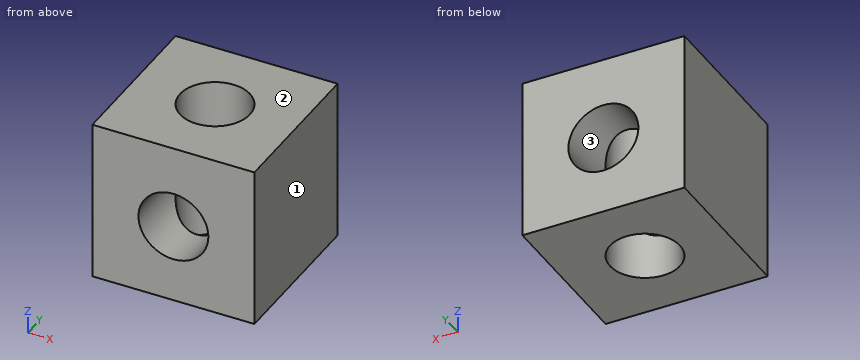
from build123d import *

# Parameters (mm, degrees)
F0_W     = 44.704
F0_H     = 44.704
F0_R     = 9.652
F1_DEPTH = 43.688
F2_R     = 9.652
F3_DEPTH = 44.705


with BuildPart() as f1:
    # F0 (on Front) → F1 (new body)
    with BuildSketch(Plane.XZ):
        with Locations((-17.125217, 3.559626)):
            Rectangle(F0_W, F0_H)
        with Locations((-17.125217, 2.924626)):
            Circle(F0_R, mode=Mode.SUBTRACT)
    extrude(amount=F1_DEPTH)

    # F2 (on face) → F3 (cut, through all)
    with BuildSketch(Plane.XY.offset(25.911626)):
        with Locations((-17.125217, -21.844)):
            Circle(F2_R)
    extrude(amount=-F3_DEPTH, mode=Mode.SUBTRACT)


solid = f1.part
Can you work these out from the model? Positions are in its coordinate system, mm. Face numbers are marked on the shaded views. Coordinates: 2 decimals unless noted, no trailing zeros. Write each loop counter-clockwise with the first axis right and the second up, starting at its lowest first coordinate (ties: lowest second). Pieces come first, ordered by that corner, then holes. Notation, with made-up numbers: (81, 85.25) - (131, 85.25) arc R28 ccw to (131, 109.25) - close; hole circle Ø11 at (60, 60). An arc over 180 degrees is marked (long way). Return JSON: item names as keys, results as strings. Group by question number.
Item 1: I'm going to push a flat-ended pin straight in: pin 1 Ø15.5 at (x, z) = (-17.13, 2.92) entering from -Y. Where does the tip first touch, or does it pass through?
Item 2: If we section it at D-D (y = -9): Write out the boundary of the cut face in (x, z), then the cut area to 3 significant figures.
Item 3: If we section it at C-C (x = -8.5): Write out the boundary of the cut face in (y, z).
Item 4: If we section it at B-B (y = -20.5): Write out the boundary of the cut face in (x, z).
Item 5: If we section it at A-A (z = 23): Write out the boundary of the cut face in (x, y), then the cut area to 3 significant figures.
Item 6: We'd pull the mould along Z, two halves only. Please class the marked faces 1, 2 and 3: pulls with the +Z half, pulls with the -Z half, needs draft (parallel to the pull), parting line crosses it, or undercut.
Item 7: Please list where these lines run through material, in increasing order: probe 1 along X at (y, z) = (-36, -6); probe 2 along Z at (x, y) = (-24.5, -39.5); probe 3 along X at (y, z) = (-30, 5.5).
Return value:
{
 "1": {"pin 1": "passes through"},
 "2": {"outline": "(-39.48, -18.79) - (5.23, -18.79) - (5.23, 25.91) - (-39.48, 25.91) - close; hole circle Ø19.3 at (-17.13, 2.92)", "area": "1,710 mm^2"},
 "3": {"outline": "(-43.69, -18.79) - (-26.18, -18.79) - (-26.18, -1.41) - (-43.69, -1.41) - close; (-43.69, 7.26) - (-26.18, 7.26) - (-26.18, 25.91) - (-43.69, 25.91) - close; (-17.51, -18.79) - (0, -18.79) - (0, -1.41) - (-17.51, -1.41) - close; (-17.51, 7.26) - (0, 7.26) - (0, 25.91) - (-17.51, 25.91) - close"},
 "4": {"outline": "(-39.48, -18.79) - (-26.68, -18.79) - (-26.68, 1.58) arc R9.65 cw to (-26.68, 4.27) - (-26.68, 25.91) - (-39.48, 25.91) - close; (-7.57, -18.79) - (5.23, -18.79) - (5.23, 25.91) - (-7.57, 25.91) - (-7.57, 4.27) arc R9.65 cw to (-7.57, 1.58) - close"},
 "5": {"outline": "(-39.48, -43.69) - (5.23, -43.69) - (5.23, 0) - (-39.48, 0) - close; hole circle Ø19.3 at (-17.13, -21.84)", "area": "1,660 mm^2"},
 "6": {"face 1": "needs draft", "face 2": "pulls with the +Z half", "face 3": "undercut"},
 "7": {"probe 1": "x = -39.48 to -20.8, -13.45 to 5.23", "probe 2": "z = -18.79 to -3.3, 9.15 to 25.91", "probe 3": "x = -39.48 to -26.43, -7.82 to 5.23"}
}
